Source: CAD feature listing. Evaluate the final solid. Frame: model axes, mm. A direction names the side the tool comes from. Give positions to 0.01 mm unless a question says otherwise; leave off trailing zeros. Order: outer loops, then holes, each group sorted by start corner. A loop starts at its lowest first (then second) coordinate and runs counter-clockwise, first axis right, second up. Notation, with made-up numbers: (7.25, 11.25) - (43.25, 11.25) arc R20 ccw to (43.25, 26.25) - close; hole circle Ø6 at (70.25, 17.25). An arc over 180 degrees is marked (long way). Write each question's results on one line, items separated by ' | '. Start each with the question number.
Item 1: Section C-C on z = -18. Output: boundary loops of the cut face in (x, y), and give its area (3 significant figures).
Item 2: Section B-B on y = 4.5. Output: boundary loops of the cut face in (x, z).
Item 3: Section A-A on z = -10. Output: boundary loops of the cut face in (x, y), and give its area (3 significant figures).
Item 4: Mould query, pull axis X, two halves, no side actions, for faces 1 (the cylindrical face through (-0.601, 24.65, -27.302)), 2 (the flat face through (7, 50, -25)), 3 (the cylindrical face through (-26.089, 24.65, 1.914)), 4 (the flat face through (-46.045, 25, 2)). Classes: released by +X, released by -X, zero draft, split by the parting line, or undercut.
Item 5: Contact query for flat-ended pins moving along their axis: pin 1 Ø20 at (x, y) = (38, 33.5) entering from -Z; pin 2 Ø10 at (x, z) = (-23, -5.5) entering from -Y; pin 3 Ø6 at (y, z) = (35, -21.5) entering from -X; pin 4 Ø2 at (y, z) = (6, -6) entering from +X. Output: stop coordinate, or through.
Item 6: Set-up query: faces 5 (the flat face through (46.045, 25, 2)), 6 (the flat face through (-37, 25, 0.737)), 7 (the cylindrical face through (26.089, 25.35, 1.914)), 8 (the flat face through (37, 25, 0.737)). Return all of +Z, -Z, +X, -X, +Y, -Y with unobstructed straight access to the full face (end or side cutting, diameter ignored); none if empty.
Item 7: Section D-D on x = 0. Output: boundary loops of the cut face in (y, z), and give its area (3 significant figures).
Item 8: Line query: line 1 along Z through (x, y) = (37.5, 27.5); line 2 along Z through (x, y) = (0.5, 41); line 3 along X through (y, z) = (33, -18). Output: solid intervals per line, ascending.
```python
from build123d import *

# Parameters (mm, degrees)
BASE_FLANGE1_DEPTH      = 50
EDGE_FLANGE1_DEPTH      = 50
EDGE_FLANGE1_BEND_DEPTH = 50


# Sheet-metal steps are written as plain solids
with BuildPart() as part:
    # Sketch1 → Base-Flange1 (new body)
    with BuildSketch(Plane(origin=(0, 0, 0), x_dir=(1, 0, 0), z_dir=(0, 1, 0))):
        with BuildLine():
            ThreePointArc((25.308741749, 0), (0, 25.308741749), (-25.308741749, 0))
            Line((-25.308741749, 0), (-27.308741749, 0))
            ThreePointArc((-27.308741749, 0), (0, 27.308741749), (27.308741749, 0))
            Line((27.308741749, 0), (25.308741749, 0))
        make_face()
    extrude(amount=BASE_FLANGE1_DEPTH)

    # Edge-Flange1 section (across the edge) → Edge-Flange1 (add)
    with BuildSketch(Plane(origin=(27.308741749, 50, 0.7366), x_dir=(0, 0, -1), z_dir=(0, -1, 0))):
        with BuildLine():
            Line((-2, 0.7366), (-2, 18.7366))
            Line((-2, 18.7366), (0, 18.7366))
            Line((0, 18.7366), (0, 0.7366))
            ThreePointArc((0, 0.7366), (0.215745145, 0.215745145), (0.7366, 0))
            Line((0.7366, 0), (0.7366, -2))
            ThreePointArc((0.7366, -2), (-1.198468417, -1.198468417), (-2, 0.7366))
        make_face()
    extrude(amount=EDGE_FLANGE1_DEPTH)

    # Edge-Flange1 section 2 (across the edge) → Edge-Flange1 bend (add)
    with BuildSketch(Plane(origin=(-27.308741749, 0, 0.7366), x_dir=(0, 0, -1), z_dir=(0, 1, 0))):
        with BuildLine():
            Line((-2, 0.7366), (-2, 18.7366))
            Line((-2, 18.7366), (0, 18.7366))
            Line((0, 18.7366), (0, 0.7366))
            ThreePointArc((0, 0.7366), (0.215745145, 0.215745145), (0.7366, 0))
            Line((0.7366, 0), (0.7366, -2))
            ThreePointArc((0.7366, -2), (-1.198468417, -1.198468417), (-2, 0.7366))
        make_face()
    extrude(amount=EDGE_FLANGE1_BEND_DEPTH)


solid = part.part
```
Evaluation:
1) outline: (-20.54, 0) - (-17.79, 0) - (-17.79, 50) - (-20.54, 50) - close; (17.79, 0) - (20.54, 0) - (20.54, 50) - (17.79, 50) - close | area: 275 mm^2
2) outline: (-46.05, 0.74) - (-28.05, 0.74) arc R0.74 cw to (-27.31, 0) arc R27.31 ccw to (27.31, 0) arc R0.74 cw to (28.05, 0.74) - (46.05, 0.74) - (46.05, 2.74) - (28.05, 2.74) arc R2.74 ccw to (25.31, 0) arc R25.31 cw to (-25.31, 0) arc R2.74 ccw to (-28.05, 2.74) - (-46.05, 2.74) - close
3) outline: (-25.41, 0) - (-23.25, 0) - (-23.25, 50) - (-25.41, 50) - close; (23.25, 0) - (25.41, 0) - (25.41, 50) - (23.25, 50) - close | area: 216 mm^2
4) face 1: split by the parting line | face 2: zero draft | face 3: undercut | face 4: released by -X
5) pin 1: stops at z = 0.74 | pin 2: stops at y = 0 | pin 3: stops at x = -20.09 | pin 4: stops at x = 26.85
6) face 5: +Z, -Z, +X, +Y, -Y | face 6: -Z, -X, +Y, -Y | face 7: +Z, +Y, -Y | face 8: -Z, +X, +Y, -Y
7) outline: (0, -27.31) - (50, -27.31) - (50, -25.31) - (0, -25.31) - close | area: 100 mm^2
8) line 1: z = 0.74 to 2.74 | line 2: z = -27.3 to -25.3 | line 3: x = -20.54 to -17.79, 17.79 to 20.54
